from build123d import *

# Parameters (mm, degrees)
F0_W     = 39.878
F0_H     = 39.878
F1_DEPTH = 9.906
F2_R     = 2.54
F3_W     = 34.798
F3_H     = 34.798
F4_DEPTH = 8.382
F5_R     = 1.042457


with BuildPart() as f1:
    # F0 (on Top) → F1 (new body)
    with BuildSketch(Plane.XY):
        with Locations((-6.466975, -3.760295)):
            Rectangle(F0_W, F0_H)
    extrude(amount=F1_DEPTH)

    # F2
    f2_edges = [f1.edges().sort_by_distance(p)[0] for p in [
        (13.472025, -23.699295, 4.953),
        (-26.405975, -23.699295, 4.953),
        (-26.405975, 16.178705, 4.953),
        (13.472025, 16.178705, 4.953),
    ]]
    fillet(f2_edges, radius=F2_R)

    # F3 (on face) → F4 (cut)
    with BuildSketch(Plane.XY.offset(9.906)):
        with Locations((-6.466975, -3.760295)):
            Rectangle(F3_W, F3_H)
    extrude(amount=-F4_DEPTH, mode=Mode.SUBTRACT)

    # F5
    f5_edges = [f1.edges().sort_by_distance(p)[0] for p in [
        (-23.865975, 13.638705, 5.715),
        (10.932025, 13.638705, 5.715),
        (10.932025, -21.159295, 5.715),
        (-23.865975, -21.159295, 5.715),
    ]]
    fillet(f5_edges, radius=F5_R)


solid = f1.part
Can you work these out from the model? Positions are in its coordinate system, mm. A direction names the side the tool comes from. Give positions to 0.01 mm unless a question says otherwise; leave off trailing zeros. Loops run counter-clockwise (first coordinate to the right, second up) from the corner with the lowest first, then second, coordinate; pieces in that order, holes last. Notation, with made-up numbers: (-20.75, -0.75) - (-1.75, -0.75) arc R6 cw to (-1.75, 9.25) - close; hole circle Ø2 at (56.5, -38.5). An arc over 180 degrees is marked (long way). Return JSON: item names as keys, results as strings.
1. I want a section at C-C on x = -14. Please give me the cut outline in (y, z), and give its area (3 significant figures).
Output values:
{"outline": "(-23.7, 0) - (16.18, 0) - (16.18, 9.91) - (13.64, 9.91) - (13.64, 1.52) - (-21.16, 1.52) - (-21.16, 9.91) - (-23.7, 9.91) - close", "area": "103 mm²"}
2. If I drill on line 1 (X direction, y = 4, z = 9.75); line 2 (Y direction, x = -16.5, z = 5.25); line 3 (Z direction, x = -16, y = -6.5), over which ranges is the centre line in solid material (lowest first)?
Output values:
{"line 1": "x = -26.41 to -23.87, 10.93 to 13.47", "line 2": "y = -23.7 to -21.16, 13.64 to 16.18", "line 3": "z = 0 to 1.52"}
3. I want a section at B-B on y = -15.5. Please give me the cut outline in (x, z), and give its area (3 significant figures).
Output values:
{"outline": "(-26.41, 0) - (13.47, 0) - (13.47, 9.91) - (10.93, 9.91) - (10.93, 1.52) - (-23.87, 1.52) - (-23.87, 9.91) - (-26.41, 9.91) - close", "area": "103 mm²"}
4. I want a section at A-A on z = 2.25. Please give me the cut outline in (x, y), and give its area (3 significant figures).
Output values:
{"outline": "(-26.41, -21.16) arc R2.54 ccw to (-23.87, -23.7) - (10.93, -23.7) arc R2.54 ccw to (13.47, -21.16) - (13.47, 13.64) arc R2.54 ccw to (10.93, 16.18) - (-23.87, 16.18) arc R2.54 ccw to (-26.41, 13.64) - close; hole (-23.87, -20.12) arc R1.04 ccw to (-22.82, -21.16) - (9.89, -21.16) arc R1.04 ccw to (10.93, -20.12) - (10.93, 12.6) arc R1.04 ccw to (9.89, 13.64) - (-22.82, 13.64) arc R1.04 ccw to (-23.87, 12.6) - close", "area": "375 mm²"}
5. For faces 5 (the face through (10.62, -20.86, 5.66)), 6 (the face through (-25.68, -22.94, 5.02)), which set-ups out of +Z, -Z, +X, -X, +Y, -Y let a thin tool reach every point of the face, with its end or its side?
Output values:
{"face 5": "+Z", "face 6": "+Z, -Z, -X, -Y"}
6. We'd pull the mould along Y, two halves only. Please class faces 1 (the face through (-7, -4, 1.524)), 2 (the face through (-7, -3, 0)), 3 (the face through (-7, -23.699, 5)), 4 (the face through (12.75, 15.41, 5.02)): +Y half, -Y half, draft (parallel to the pull), parting line (faces both ways), or undercut.
Output values:
{"face 1": "undercut", "face 2": "draft", "face 3": "-Y half", "face 4": "+Y half"}
7. I'm going to push a flat-ended pin straight in: pin 1 Ø17.5 at (x, y) = (-10, 1.5) entering from +Z. Where does the tip first touch, or does it pass through?
Output values:
{"pin 1": "stops at z = 1.52"}
